For this review, take the finished solid that the model builds, in its own axes (mm). A direction names the side the tool comes from. Round coordinates to 2 decimals unless told otherwise and drop trailing zeros. Loops run counter-clockwise (first coordinate to the right, second up) from the corner with the lowest first, then second, coordinate; pieces in that order, holes last.
1. Draft analysis for pull direction X (two halves, no side actions). For faces 1 (the flat face through (-13.51, -3.13, 3.72)), 2 (the flat face through (6.879, -3.131, -12.165)), 3 (the flat face through (13.873, -3.131, 1.971)), state which applies: released by +X, released by -X, zero draft, split by the parting line, or undercut.
2. To check wall thickness, follow line 1 along Z through (x, y) = (-12, -4.5); line 2 along X through (y, z) = (-6, -13); line 3 along X through (y, z) = (-3.25, -12). State the ranges of each line that lie inside material, in increasing order.
3. Clearance check with flat-ended pins moving along their axes: pin 1 Ø1.5 at (y, z) = (-1, -10) entering from -X; pin 2 Ø12 at (x, z) = (-7, 7) entering from +Y; pin 3 Ø1 at (y, z) = (-3, 9) entering from +X. State where each tip first meets the part, or that it passes through.
4. Tool access review of faces 4 (the flat face through (13.89, -3.131, -1.845)), 5 (the flat face through (5.972, -3.131, 12.635)), 6 (the flat face through (-9.61, -3.13, 10.2)): name each direction out of +Z, -Z, +X, -X, +Y, -Y from which nothing blocks a thin tool from reaching the whole face with its end or side.
5. Consider section A-A on x = 4. State the section outline as (y, z) points.
from build123d import *

# Parameters (mm, degrees)
F0_R     = 2.159
F1_DEPTH = 6.35


with BuildPart() as f1:
    # F0 (on Front) → F1 (new body)
    with BuildSketch(Plane.XZ):
        with BuildLine():
            ThreePointArc((12.695722, -0.329596), (12.698931, -0.164812), (12.7, 0))
            ThreePointArc((12.7, 0), (12.633417, 1.298755), (12.434368, 2.583891))
            ThreePointArc((12.434368, 2.583891), (12.376885, 2.846529), (12.313854, 3.107891))
            ThreePointArc((12.313854, 3.107891), (11.874003, 4.505335), (11.276142, 5.842826))
            ThreePointArc((11.276142, 5.842826), (11.149932, 6.080216), (11.018724, 6.31488))
            ThreePointArc((11.018724, 6.31488), (10.218158, 7.541833), (9.281617, 8.668425))
            ThreePointArc((9.281617, 8.668425), (9.09604, 8.86296), (8.906386, 9.053524))
            ThreePointArc((8.906386, 9.053524), (7.804479, 10.018987), (6.598716, 10.851126))
            ThreePointArc((6.598716, 10.851126), (6.367536, 10.98838), (6.133501, 11.120709))
            ThreePointArc((6.133501, 11.120709), (4.811977, 11.753079), (3.426419, 12.22905))
            ThreePointArc((3.426419, 12.22905), (3.166781, 12.298841), (2.905723, 12.363121))
            ThreePointArc((2.905723, 12.363121), (1.462593, 12.615499), (0, 12.7))
            ThreePointArc((0, 12.7), (-0.26884, 12.697154), (-0.537559, 12.688618))
            ThreePointArc((-0.537559, 12.688618), (-1.995265, 12.542285), (-3.426419, 12.22905))
            ThreePointArc((-3.426419, 12.22905), (-3.684522, 12.153777), (-3.940973, 12.073058))
            ThreePointArc((-3.940973, 12.073058), (-5.305143, 11.538867), (-6.598716, 10.851126))
            ThreePointArc((-6.598716, 10.851126), (-6.826939, 10.70901), (-7.052103, 10.562095))
            ThreePointArc((-7.052103, 10.562095), (-8.221563, 9.679664), (-9.281617, 8.668425))
            ThreePointArc((-9.281617, 8.668425), (-9.463034, 8.470005), (-9.640211, 8.267789))
            ThreePointArc((-9.640211, 8.267789), (-10.528227, 7.102565), (-11.276142, 5.842826))
            ThreePointArc((-11.276142, 5.842826), (-11.397299, 5.602818), (-11.513349, 5.360299))
            ThreePointArc((-11.513349, 5.360299), (-12.054061, 3.998701), (-12.434368, 2.583891))
            ThreePointArc((-12.434368, 2.583891), (-12.486279, 2.320096), (-12.532594, 2.05526))
            ThreePointArc((-12.532594, 2.05526), (-12.6859, 0.598271), (-12.670393, -0.866679))
            ThreePointArc((-12.670393, -0.866679), (-12.649208, -1.134697), (-12.622354, -1.402208))
            ThreePointArc((-12.622354, -1.402208), (-12.376885, -2.846529), (-11.966714, -4.252971))
            ThreePointArc((-11.966714, -4.252971), (-11.874003, -4.505335), (-11.775971, -4.75568))
            ThreePointArc((-11.775971, -4.75568), (-11.149932, -6.080216), (-10.375518, -7.32384))
            ThreePointArc((-10.375518, -7.32384), (-10.218158, -7.541833), (-10.056219, -7.756446))
            ThreePointArc((-10.056219, -7.756446), (-9.09604, -8.86296), (-8.014817, -9.851533))
            ThreePointArc((-8.014817, -9.851533), (-7.804479, -10.018987), (-7.590643, -10.181951))
            ThreePointArc((-7.590643, -10.181951), (-6.367536, -10.98838), (-5.059694, -11.648584))
            ThreePointArc((-5.059694, -11.648584), (-4.811977, -11.753079), (-4.562104, -11.852308))
            ThreePointArc((-4.562104, -11.852308), (-3.166781, -12.298841), (-1.729316, -12.581712))
            ThreePointArc((-1.729316, -12.581712), (-1.462593, -12.615499), (-1.195214, -12.643633))
            ThreePointArc((-1.195214, -12.643633), (0.26884, -12.697154), (1.729316, -12.581712))
            ThreePointArc((1.729316, -12.581712), (1.995265, -12.542285), (2.260319, -12.497238))
            ThreePointArc((2.260319, -12.497238), (3.684522, -12.153777), (5.059694, -11.648584))
            ThreePointArc((5.059694, -11.648584), (5.305143, -11.538867), (5.548215, -11.42398))
            ThreePointArc((5.548215, -11.42398), (6.826939, -10.70901), (8.014817, -9.851533))
            ThreePointArc((8.014817, -9.851533), (8.221563, -9.679664), (8.424625, -9.503457))
            ThreePointArc((8.424625, -9.503457), (9.463034, -8.470005), (10.375518, -7.32384))
            ThreePointArc((10.375518, -7.32384), (10.528227, -7.102565), (10.676219, -6.878107))
            ThreePointArc((10.676219, -6.878107), (11.397299, -5.602818), (11.966714, -4.252971))
            ThreePointArc((11.966714, -4.252971), (12.054061, -3.998701), (12.136007, -3.742639))
            ThreePointArc((12.136007, -3.742639), (12.486279, -2.320096), (12.670393, -0.866679))
            ThreePointArc((12.670393, -0.866679), (12.6859, -0.598271), (12.695722, -0.329596))
        make_face()
        Circle(F0_R, mode=Mode.SUBTRACT)
        with BuildLine():
            ThreePointArc((-12.670393, -0.866679), (-12.6859, 0.598271), (-12.532594, 2.05526))
            Line((-12.532594, 2.05526), (-15.316746, 0.717239))
            Line((-15.316746, 0.717239), (-12.670393, -0.866679))
        make_face()
        with BuildLine():
            ThreePointArc((-12.434368, 2.583891), (-12.054061, 3.998701), (-11.513349, 5.360299))
            Line((-11.513349, 5.360299), (-14.555251, 4.82305))
            Line((-14.555251, 4.82305), (-12.434368, 2.583891))
        make_face()
        with BuildLine():
            ThreePointArc((-11.276142, 5.842826), (-10.528227, 7.102565), (-9.640211, 8.267789))
            Line((-9.640211, 8.267789), (-12.714259, 8.571158))
            Line((-12.714259, 8.571158), (-11.276142, 5.842826))
        make_face()
        with BuildLine():
            ThreePointArc((-9.281617, 8.668425), (-8.221563, 9.679664), (-7.052103, 10.562095))
            Line((-7.052103, 10.562095), (-9.930309, 11.683582))
            Line((-9.930309, 11.683582), (-9.281617, 8.668425))
        make_face()
        with BuildLine():
            ThreePointArc((-6.598716, 10.851126), (-5.305143, 11.538867), (-3.940973, 12.073058))
            Line((-3.940973, 12.073058), (-6.409874, 13.929489))
            Line((-6.409874, 13.929489), (-6.598716, 10.851126))
        make_face()
        with BuildLine():
            ThreePointArc((-3.426419, 12.22905), (-1.995265, 12.542285), (-0.537559, 12.688618))
            Line((-0.537559, 12.688618), (-2.414047, 15.142308))
            Line((-2.414047, 15.142308), (-3.426419, 12.22905))
        make_face()
        with BuildLine():
            ThreePointArc((0, 12.7), (1.462593, 12.615499), (2.905723, 12.363121))
            Line((2.905723, 12.363121), (1.760818, 15.232093))
            Line((1.760818, 15.232093), (0, 12.7))
        make_face()
        with BuildLine():
            ThreePointArc((3.426419, 12.22905), (4.811977, 11.753079), (6.133501, 11.120709))
            Line((6.133501, 11.120709), (5.805092, 14.192182))
            Line((5.805092, 14.192182), (3.426419, 12.22905))
        make_face()
        with BuildLine():
            ThreePointArc((6.598716, 10.851126), (7.804479, 10.018987), (8.906386, 9.053524))
            Line((8.906386, 9.053524), (9.418828, 12.099703))
            Line((9.418828, 12.099703), (6.598716, 10.851126))
        make_face()
        with BuildLine():
            ThreePointArc((9.281617, 8.668425), (10.218158, 7.541833), (11.018724, 6.31488))
            Line((11.018724, 6.31488), (12.334013, 9.109843))
            Line((12.334013, 9.109843), (9.281617, 8.668425))
        make_face()
        with BuildLine():
            ThreePointArc((11.276142, 5.842826), (11.874003, 4.505335), (12.313854, 3.107891))
            Line((12.313854, 3.107891), (14.334441, 5.444349))
            Line((14.334441, 5.444349), (11.276142, 5.842826))
        make_face()
        with BuildLine():
            ThreePointArc((12.434368, 2.583891), (12.633417, 1.298755), (12.7, 0))
            ThreePointArc((12.7, 0), (12.698931, -0.164812), (12.695722, -0.329596))
            Line((12.695722, -0.329596), (15.271749, 1.375072))
            Line((15.271749, 1.375072), (12.434368, 2.583891))
        make_face()
        with BuildLine():
            Line((15.076421, -2.796188), (12.670393, -0.866679))
            ThreePointArc((12.670393, -0.866679), (12.486279, -2.320096), (12.136007, -3.742639))
            Line((12.136007, -3.742639), (15.076421, -2.796188))
        make_face()
        with BuildLine():
            Line((13.762944, -6.760068), (11.966714, -4.252971))
            ThreePointArc((11.966714, -4.252971), (11.397299, -5.602818), (10.676219, -6.878107))
            Line((10.676219, -6.878107), (13.762944, -6.760068))
        make_face()
        with BuildLine():
            Line((11.428732, -10.222584), (10.375518, -7.32384))
            ThreePointArc((10.375518, -7.32384), (9.463034, -8.470005), (8.424625, -9.503457))
            Line((8.424625, -9.503457), (11.428732, -10.222584))
        make_face()
        with BuildLine():
            Line((8.246903, -12.926937), (8.014817, -9.851533))
            ThreePointArc((8.014817, -9.851533), (6.826939, -10.70901), (5.548215, -11.42398))
            Line((5.548215, -11.42398), (8.246903, -12.926937))
        make_face()
        with BuildLine():
            Line((4.45344, -14.672559), (5.059694, -11.648584))
            ThreePointArc((5.059694, -11.648584), (3.684522, -12.153777), (2.260319, -12.497238))
            Line((2.260319, -12.497238), (4.45344, -14.672559))
        make_face()
        with BuildLine():
            Line((0.329685, -15.329985), (1.729316, -12.581712))
            ThreePointArc((1.729316, -12.581712), (0.26884, -12.697154), (-1.195214, -12.643633))
            Line((-1.195214, -12.643633), (0.329685, -15.329985))
        make_face()
        with BuildLine():
            Line((-3.818521, -14.850455), (-1.729316, -12.581712))
            ThreePointArc((-1.729316, -12.581712), (-3.166781, -12.298841), (-4.562104, -11.852308))
            Line((-4.562104, -11.852308), (-3.818521, -14.850455))
        make_face()
        with BuildLine():
            Line((-7.683525, -13.269536), (-5.059694, -11.648584))
            ThreePointArc((-5.059694, -11.648584), (-6.367536, -10.98838), (-7.590643, -10.181951))
            Line((-7.590643, -10.181951), (-7.683525, -13.269536))
        make_face()
        with BuildLine():
            Line((-10.978677, -10.704475), (-8.014817, -9.851533))
            ThreePointArc((-8.014817, -9.851533), (-9.09604, -8.86296), (-10.056219, -7.756446))
            Line((-10.056219, -7.756446), (-10.978677, -10.704475))
        make_face()
        with BuildLine():
            Line((-13.45959, -7.345513), (-10.375518, -7.32384))
            ThreePointArc((-10.375518, -7.32384), (-11.149932, -6.080216), (-11.775971, -4.75568))
            Line((-11.775971, -4.75568), (-13.45959, -7.345513))
        make_face()
        with BuildLine():
            Line((-14.942268, -3.441767), (-11.966714, -4.252971))
            ThreePointArc((-11.966714, -4.252971), (-12.376885, -2.846529), (-12.622354, -1.402208))
            Line((-12.622354, -1.402208), (-14.942268, -3.441767))
        make_face()
    extrude(amount=F1_DEPTH)


solid = f1.part
Resolved:
1. face 1: released by -X
1. face 2: undercut
1. face 3: released by +X
2. line 1: z = -7.34 to -5.1, -4.24 to 5.27, 7.22 to 8.5
2. line 2: x = -7.68 to -7.25, -4.28 to -2.11, -0.99 to 1.52, 2.77 to 4.79
2. line 3: x = -7.65 to -5.63, -4.53 to 4.99, 6.58 to 8.18
3. pin 1: stops at x = -10.98
3. pin 2: stops at y = 0
3. pin 3: stops at x = 12.33
4. face 4: +X, +Y, -Y
4. face 5: +Z, +Y, -Y
4. face 6: -X, +Y, -Y
5. outline: (-6.35, -14.22) - (0, -14.22) - (0, 12.7) - (-6.35, 12.7) - close
